Can you work these out from the model? Positions are in its coordinate system, mm. Face numbers are marked on the shaded views. A direction names the side the tool comes from. Round coordinates to 2 decimals unless told otherwise and drop trailing zeros. Loops run counter-clockwise (first coordinate to the right, second up) from the corner with the lowest first, then second, coordinate; pieces in that order, holes last. Notation, with made-up numbers: M 87.5,12 L 95.5,12 A15 cw 95.5,22 Z; hole C -33,69 d4. An arc over 180 degrees is marked long. Use a Markdown table: item, result. Add a question column.
```python
from build123d import *

# Parameters (mm, degrees)
SKETCH2_W           = 45
SKETCH2_H           = 10
BOSS_EXTRUDE1_DEPTH = 40
SKETCH4_W           = 45
SKETCH4_H           = 10
BOSS_EXTRUDE2_DEPTH = 10
SKETCH8_W           = 45
SKETCH8_H           = 10
BOSS_EXTRUDE3_DEPTH = 20
SKETCH9_R           = 1.45
CUT_EXTRUDE2_DEPTH  = 20
SKETCH10_W          = 45
SKETCH10_H          = 0.626165357
CUT_EXTRUDE3_DEPTH  = 2
SKETCH11_W          = 19
SKETCH11_H          = 42.671327575
BOSS_EXTRUDE4_DEPTH = 1.5
SKETCH12_W          = 3
SKETCH12_H          = 27.286335608
CUT_EXTRUDE6_DEPTH  = 10
SKETCH13_W          = 13
SKETCH13_H          = 22
BOSS_EXTRUDE5_DEPTH = 1


with BuildPart() as part:
    # Sketch2 → Boss-Extrude1 (new body)
    with BuildSketch(Plane(origin=(0, 0, 0), x_dir=(1, 0, 0), z_dir=(0, 1, 0))):
        Rectangle(SKETCH2_W, SKETCH2_H)
    extrude(amount=BOSS_EXTRUDE1_DEPTH)

    # Sketch4 → Boss-Extrude2 (add)
    with BuildSketch(Plane(origin=(0, 40, 0), x_dir=(1, 0, 0), z_dir=(0, 1, 0))):
        Rectangle(SKETCH4_W, SKETCH4_H)
    extrude(amount=BOSS_EXTRUDE2_DEPTH)

    # Sketch8 → Boss-Extrude3 (add)
    with BuildSketch(Plane.XZ):
        Rectangle(SKETCH8_W, SKETCH8_H)
    extrude(amount=BOSS_EXTRUDE3_DEPTH)

    # Sketch9 → Cut-Extrude2 (cut)
    with BuildSketch(Plane.XY.offset(5)):
        with Locations((19.5, 11.5)):
            Circle(SKETCH9_R)
        with Locations((-19.5, 11.5)):
            Circle(SKETCH9_R)
    extrude(amount=-CUT_EXTRUDE2_DEPTH, mode=Mode.SUBTRACT)

    # Sketch10 → Cut-Extrude3 (cut)
    with BuildSketch(Plane.XY.offset(5)):
        with Locations((0, 22.984410254)):
            Rectangle(SKETCH10_W, SKETCH10_H)
    extrude(amount=-CUT_EXTRUDE3_DEPTH, mode=Mode.SUBTRACT)

    # Sketch11 → Boss-Extrude4 (add)
    with BuildSketch(Plane.XY.offset(5)):
        with Locations((0, 1.335663788)):
            Rectangle(SKETCH11_W, SKETCH11_H)
    extrude(amount=BOSS_EXTRUDE4_DEPTH)

    # Sketch12 → Cut-Extrude6 (cut)
    with BuildSketch(Plane(origin=(22.5, 0, 0), x_dir=(0, 0, -1), z_dir=(1, 0, 0))):
        with Locations((0, -4.971840229)):
            Rectangle(SKETCH12_W, SKETCH12_H)
    extrude(amount=-CUT_EXTRUDE6_DEPTH, mode=Mode.SUBTRACT)

    # Sketch13 → Boss-Extrude5 (add)
    with BuildSketch(Plane.XY.offset(5)):
        with Locations((16, -9)):
            Rectangle(SKETCH13_W, SKETCH13_H)
    extrude(amount=BOSS_EXTRUDE5_DEPTH)


solid = part.part
```
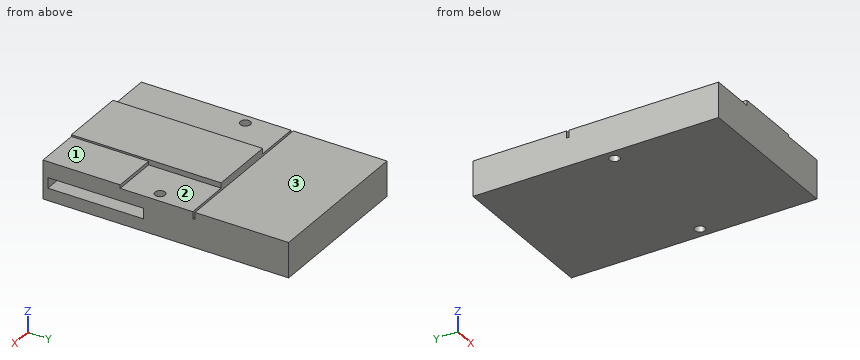
(1) Suppose I cut it at C-C on x = 14.5. List the corners of the cut face in (y, z) for me (1 decimal).
(2) I'm going to push flat-ended pins straight in: pin 1 (4 mm diameter, centred on x = 1.5, z = 5.5, fed in from +Y); pin 2 (3.5 mm diameter, centred on x = 19.5, y = 11.5, fed in from +Z); pin 3 (0.8 mm diameter, centred on y = 5, z = 5.5, fed in from +X); pin 4 (0.9 mm diameter, centred on y = -8.5, z = -0.5, fed in from +X). Where does each tip first touch, or does it pass through?
(3) Suppose I cut it at B-B on x = 19.5. Count the separate pieces of the cut face and the enclosed holes in it, and give its area (3 significant figures).
(4) On a 3-axis mill with a long thin cutter (end or side, diameter ignored), from which of +Z, -Z, +X, -X, +Y, -Y can I reach the whole of each face in a straight line? I mean the marked faces 1, 2 and 3. Say none if no direction works.
(5) Suppose I cut it at A-A on y = 11.5. List the corners of the cut face in (x, z) for me.
(6) Suppose I cut it at D-D on z = 0.75. List the corners of the cut face in (x, y) for me (3 decimals).
(7) If I drill on probe 1 along Y at (x, z) = (19.5, 2.25); probe 2 along Z at (x, y) = (17, -5.5); probe 3 along Y at (x, z) = (13, 3.25), over which ranges is the centre line in solid material (lowest first)? Write a range as [from, to].
Results below:
| question | item | result |
|---|---|---|
| 1 | outline | M -20,-5 L 50,-5 L 50,5 L 23.3,5 L 23.3,3 L 22.7,3 L 22.7,5 L 2,5 L 2,6 L -20,6 Z; hole M -18.6,-1.5 L 8.7,-1.5 L 8.7,1.5 L -18.6,1.5 Z |
| 2 | pin 1 | stops at y = 50 |
| 2 | pin 2 | stops at z = 5 |
| 2 | pin 3 | stops at x = 9.5 |
| 2 | pin 4 | stops at x = 12.5 |
| 3 | separate pieces | 2 |
| 3 | enclosed holes | 1 |
| 3 | area | 610 mm² |
| 4 | face 1 | +Z, +X, +Y, -Y |
| 4 | face 2 | +Z, +X, +Y |
| 4 | face 3 | +Z, +X, -X, +Y |
| 5 | outline | M -22.5,-5 L -20.95,-5 L -20.95,5 L -22.5,5 Z; M -18.05,-5 L 18.05,-5 L 18.05,5 L 9.5,5 L 9.5,6.5 L -9.5,6.5 L -9.5,5 L -18.05,5 Z; M 20.95,-5 L 22.5,-5 L 22.5,5 L 20.95,5 Z |
| 6 | outline | M -22.5,-20 L 22.5,-20 L 22.5,-18.615 L 12.5,-18.615 L 12.5,8.671 L 22.5,8.671 L 22.5,50 L -22.5,50 Z; hole C -19.5,11.5 d2.9; hole C 19.5,11.5 d2.9 |
| 7 | probe 1 | y = [-20, 10.05], [12.95, 50] |
| 7 | probe 2 | z = [-5, -1.5], [1.5, 6] |
| 7 | probe 3 | y = [-20, 22.67], [23.3, 50] |
